from build123d import *

# Parameters (mm, degrees)
SKETCH_1_R          = 18
EXTRUDE_3_DEPTH     = 9
SKETCH_4_R          = 16
CUT_EXTRUDE_1_DEPTH = 4
SKETCH_5_R          = 15
CUT_EXTRUDE_2_DEPTH = 0.5
SKETCH_7_R          = 9
CUT_EXTRUDE_3_DEPTH = 26.850531909
SKETCH_11_R         = 23
SKETCH_11_R_2       = 18
EXTRUDE_4_DEPTH     = 3
CHAMFER_2_SIZE      = 0.5
HOLE_WIZARD_M3_2_D  = 2.5


with BuildPart() as part:
    # 草图1 → 凸台-拉伸3 (new body)
    with BuildSketch(Plane.XY):
        Circle(SKETCH_1_R)
    extrude(amount=EXTRUDE_3_DEPTH)

    # 草图4 → 切除-拉伸1 (cut)
    with BuildSketch(Plane.XY.offset(9)):
        Circle(SKETCH_4_R)
    extrude(amount=-CUT_EXTRUDE_1_DEPTH, mode=Mode.SUBTRACT)

    # 草图5 → 切除-拉伸2 (cut)
    with BuildSketch(Plane.XY.offset(5)):
        Circle(SKETCH_5_R)
    extrude(amount=-CUT_EXTRUDE_2_DEPTH, mode=Mode.SUBTRACT)

    # 草图7 → 切除-拉伸3 (cut, through all)
    with BuildSketch(Plane.XY.offset(4.5)):
        Circle(SKETCH_7_R)
    extrude(amount=-CUT_EXTRUDE_3_DEPTH, mode=Mode.SUBTRACT)

    # 草图11 → 凸台-拉伸4 (add)
    with BuildSketch(Plane(origin=(0, 0, 0), x_dir=(-1, 0, 0), z_dir=(0, 0, -1))):
        Circle(SKETCH_11_R)
        Circle(SKETCH_11_R_2, mode=Mode.SUBTRACT)
    extrude(amount=-EXTRUDE_4_DEPTH)

    # 倒角2
    chamfer_2_edges = [part.edges().sort_by_distance(p)[0] for p in [
        (-9, 0, 0),
    ]]
    chamfer(chamfer_2_edges, length=CHAMFER_2_SIZE)

    # M3 螺纹孔2 (through all)
    with Locations(Plane(origin=(0, 0, 0), x_dir=(-1, 0, 0), z_dir=(0, 0, -1))):
        with Locations((0, 20), (-20, 0), (0, -20), (20, 0)):
            Hole(HOLE_WIZARD_M3_2_D / 2)


solid = part.part
Geometry: final body of the model. Coordinates: model frame, mm. A direction names the side the tool comes from. Give positions to 0.01 mm unless a question says otherwise; leave off trailing zeros. Order: outer loops, then holes, each group sorted by start corner. A loop starts at its lowest first (then second) coordinate and runs counter-clockwise, first axis right, second up. Notation, with made-up numbers: (3, -19) -> (41, -19) arc R26 cw to (41, 11) -> close; hole circle Ø4 at (17, 12.25). An arc over 180 degrees is marked (long way). Write each question's results on one line, items separated by ' | '.
1) Draft query along Y for faces 1 (the face through (2.994, 22.804, 1.479)), 2 (the face through (21.155, -0.479, 1.521)), 3 (the face through (-12, -11, 9)). Return one class per face: released by +Y, released by -Y, zero draft, split by the parting line, or undercut.
Geometry says:
face 1: split by the parting line | face 2: undercut | face 3: zero draft
2) Cut plane A-A (x = 0). Give the number of separate pieces and of enclosed holes in the cut face, and give its area (3 significant figures).
Geometry says:
separate pieces: 4 | enclosed holes: 0 | area: 115 mm²
3) Line query: line 1 along Y through (x, z) = (0, 1.8); line 2 along Z through (x, y) = (10, 20); line 3 along Z through (x, y) = (-13.5, -8). Output: solid intervals per line, ascending.
Geometry says:
line 1: y = -23 to -21.25, -18.75 to -9, 9 to 18.75, 21.25 to 23 | line 2: z = 0 to 3 | line 3: z = 0 to 5
4) Set-up query: faces 4 (the face through (-0.27, -21.22, 1.52)), 5 (the face through (6.5, -6.5, 4.5)). Return all of +Z, -Z, +X, -X, +Y, -Y with unobstructed straight access to the full face (end or side cutting, diameter ignored); none if empty.
Geometry says:
face 4: +Z, -Z | face 5: +Z
5) Cut plane D-D (x = -20). Output: boundary loops of the cut face in (y, z), and give its area (3 significant figures).
Geometry says:
outline: (-11.36, 0) -> (-1.25, 0) -> (-1.25, 3) -> (-11.36, 3) -> close; (1.25, 0) -> (11.36, 0) -> (11.36, 3) -> (1.25, 3) -> close | area: 60.6 mm²
6) Cut plane C-C (z = 2.25). Output: boundary loops of the cut face in (x, y).
Geometry says:
outline: circle Ø46 at (0, 0); hole circle Ø2.5 at (-20, 0); hole circle Ø18 at (0, 0); hole circle Ø2.5 at (0, -20); hole circle Ø2.5 at (0, 20); hole circle Ø2.5 at (20, 0)
7) First-contact query: pin 1 Ø1.5 at (x, z) = (4, 4.5) entering from +Y; pin 2 Ø5 at (x, y) = (5.5, -2) entering from -Z (3 decimals); pin 3 Ø9 at (x, y) = (-5.5, 5.5) entering from +Z; pin 4 Ø1 at (y, z) = (3.5, 2.5) entering from +X. Flat tips, straight axial feed; report the tip coordinate or a pass-through.
Geometry says:
pin 1: stops at y = 17.7 | pin 2: passes through | pin 3: stops at z = 4.5 | pin 4: stops at x = 22.8
